```python
from build123d import *

# Parameters (mm, degrees)
COMPONENT_OUTLINE_W = 9.8
COMPONENT_OUTLINE_H = 4.1
EXTRUDE1_DEPTH      = 8
CUT_EXTRUDE1_DEPTH  = 5
SKETCH3_R           = 0.5
CUT_EXTRUDE2_DEPTH  = 5
SKETCH4_R           = 1.5
CUT_EXTRUDE3_DEPTH  = 0.1


with BuildPart() as part:
    # COMPONENT_OUTLINE → Extrude1 (new body)
    with BuildSketch(Plane.XY):
        with Locations((0, -3.45)):
            Rectangle(COMPONENT_OUTLINE_W, COMPONENT_OUTLINE_H)
    extrude(amount=EXTRUDE1_DEPTH)

    # Sketch1 → Cut-Extrude1 (cut)
    with BuildSketch(Plane.XY.offset(8)):
        with BuildLine():
            Line((0.798435971, -5.5), (4.9, -5.5))
            Line((4.9, -5.5), (4.9, -1.4))
            Line((4.9, -1.4), (0.798435971, -1.4))
            ThreePointArc((0.798435971, -1.4), (2.2, -3.45), (0.798435971, -5.5))
        make_face()
        with BuildLine():
            Line((-0.798435971, -1.4), (-4.9, -1.4))
            Line((-4.9, -1.4), (-4.9, -5.5))
            Line((-4.9, -5.5), (-0.798435971, -5.5))
            ThreePointArc((-0.798435971, -5.5), (-2.2, -3.45), (-0.798435971, -1.4))
        make_face()
    extrude(amount=-CUT_EXTRUDE1_DEPTH, mode=Mode.SUBTRACT)

    # Sketch3 → Cut-Extrude2 (cut)
    with BuildSketch(Plane.XY.offset(8)):
        with Locations((0, -3.45)):
            Circle(SKETCH3_R)
    extrude(amount=-CUT_EXTRUDE2_DEPTH, mode=Mode.SUBTRACT)

    # Sketch4 → Cut-Extrude3 (cut)
    with BuildSketch(Plane.XY.offset(8)):
        with Locations((0, -3.45)):
            Circle(SKETCH4_R)
    extrude(amount=-CUT_EXTRUDE3_DEPTH, mode=Mode.SUBTRACT)


solid = part.part
```
Can you work these out from the model? Positions are in its coordinate system, mm. A direction names the side the tool comes from. Coordinates: 2 decimals unless noted, no trailing zeros. Order: outer loops, then holes, each group sorted by start corner. A loop starts at its lowest first (then second) coordinate and runs counter-clockwise, first axis right, second up.
1. If we section it at C-C (x = 0): Please give me the cut outline in (y, z).
2. If we section it at A-A (z = 7.75): Please give me the cut outline in (x, y), then the cut area to 3 significant figures.
3. I'm going to push flat-ended pins straight in: pin 1 (1.1 mm diameter, centred on x = 0, y = -3.5, fed in from +Z); pin 2 (2 mm diameter, centred on x = -3.5, y = -4.5, fed in from +Z); pin 3 (4 mm diameter, centred on x = -3.5, z = 6.5, fed in from -Y). Where does each tip first touch, or does it pass through?
4. For faces 4 (the face through (2.2, -3.4, 5.5)), 5 (the face through (0, -3.4, 3)), 6 (the face through (-4.9, -3, 1)), which set-ups out of +Z, -Z, +X, -X, +Y, -Y let a thin tool reach every point of the face, with its end or its side?
5. If we section it at D-D (y = -4.45): Please give me the cut outline in (x, z), then the cut area to 3 significant figures.
6. Thinking about a two-plate mould opening in Y: for faces 1 (the face through (-0.02, -4.1, 7.9)), 2 (the face through (0, -3, 0)), 3 (the face through (-2.2, -3.5, 5.5)), which applies, +Y half, -Y half, draft (parallel to the pull), parting line (faces both ways), or undercut?
7. If we section it at B-B (y = -3.45): Please give me the cut outline in (x, z).
8. I need wall thicknesses on line 1 (X direction, y = -3.5, z = 4); line 2 (Y direction, x = 0, z = 6.6); line 3 (Z direction, x = 1, y = -2.85). Which ranges of each line are inside material? Lowest first, please.
Entries:
1. outline: (-5.5, 0) - (-1.4, 0) - (-1.4, 8) - (-1.95, 8) - (-1.95, 7.9) - (-2.95, 7.9) - (-2.95, 3) - (-3.95, 3) - (-3.95, 7.9) - (-4.95, 7.9) - (-4.95, 8) - (-5.5, 8) - close
2. outline: (-0.8, -5.5) - (0.8, -5.5) arc R2.2 ccw to (0.8, -1.4) - (-0.8, -1.4) arc R2.2 ccw to start; hole circle Ø1 at (0, -3.45)
2. area: 14.1 mm2
3. pin 1: stops at z = 7.9
3. pin 2: stops at z = 3
3. pin 3: stops at y = -5.06
4. face 4: +Z, +X
4. face 5: +Z
4. face 6: +Z, -Z, -X, +Y, -Y
5. outline: (-4.9, 0) - (4.9, 0) - (4.9, 3) - (1.96, 3) - (1.96, 8) - (1.12, 8) - (1.12, 7.9) - (-1.12, 7.9) - (-1.12, 8) - (-1.96, 8) - (-1.96, 3) - (-4.9, 3) - close
5. area: 48.8 mm2
6. face 1: undercut
6. face 2: draft
6. face 3: parting line
7. outline: (-4.9, 0) - (4.9, 0) - (4.9, 3) - (2.2, 3) - (2.2, 8) - (1.5, 8) - (1.5, 7.9) - (0.5, 7.9) - (0.5, 3) - (-0.5, 3) - (-0.5, 7.9) - (-1.5, 7.9) - (-1.5, 8) - (-2.2, 8) - (-2.2, 3) - (-4.9, 3) - close
8. line 1: x = -2.2 to -0.5, 0.5 to 2.2
8. line 2: y = -5.5 to -3.95, -2.95 to -1.4
8. line 3: z = 0 to 7.9
